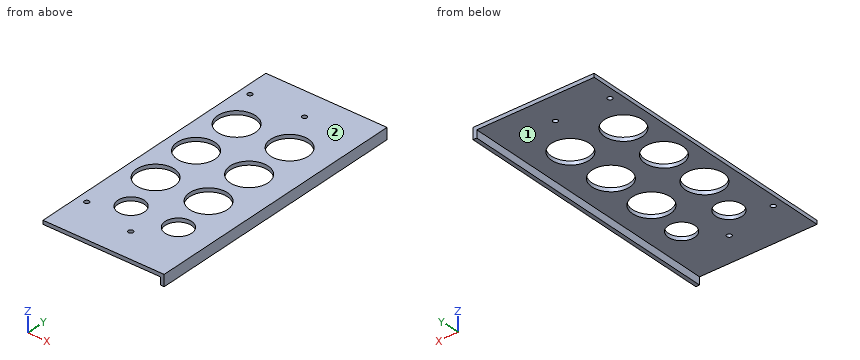
from build123d import *

# Parameters (mm, degrees)
SKETCH138_R           = 7
SKETCH138_R_2         = 10
EXTRUDE128_DEPTH      = 1
EXTRUDE128_DEPTH_BACK = 3
SKETCH117_R           = 1.28
EXTRUDE107_DEPTH      = 3
EXTRUDE104_DEPTH      = 143


with BuildPart() as extrude128:
    # Sketch138 → Extrude128 (new body, two sides)
    with BuildSketch(Plane(origin=(0, 0, -2), x_dir=(1, 0, 0), z_dir=(0, 0, -1))) as extrude128_sk:
        with Locations((28, -97)):
            Circle(SKETCH138_R)
        with Locations((53, -97)):
            Circle(SKETCH138_R)
        with Locations((22, -146)):
            Circle(SKETCH138_R_2)
        with Locations((50, -146)):
            Circle(SKETCH138_R_2)
        with Locations((22, -172)):
            Circle(SKETCH138_R_2)
        with Locations((50, -172)):
            Circle(SKETCH138_R_2)
        with Locations((22, -120)):
            Circle(SKETCH138_R_2)
        with Locations((50, -120)):
            Circle(SKETCH138_R_2)
    extrude(amount=EXTRUDE128_DEPTH)
    extrude(extrude128_sk.sketch, amount=-EXTRUDE128_DEPTH_BACK)


with BuildPart() as compound022:
    # Sketch117 → Extrude107 (new body)
    with BuildSketch(Plane(origin=(0, 0, 1), x_dir=(1, 0, 0), z_dir=(0, 0, -1))):
        with Locations((12, -88)):
            Circle(SKETCH117_R)
        with Locations((40, -82.25)):
            Circle(SKETCH117_R)
        with Locations((12, -192.75)):
            Circle(SKETCH117_R)
        with Locations((40, -193.75)):
            Circle(SKETCH117_R)
    extrude(amount=EXTRUDE107_DEPTH)

    # Compound022: union Extrude128
    add(extrude128.part)


with BuildPart() as hdmi002:
    # Sketch114 → Extrude104 (new body)
    with BuildSketch(Plane(origin=(0, 66, 0), x_dir=(-1, 0, 0), z_dir=(0, 1, 0))):
        Polygon((-7, -2), (-7, 0), (-71, 0), (-71, -6), (-69, -6), (-69, -2), align=None)
    extrude(amount=EXTRUDE104_DEPTH)

    # Cut013: cut Compound022
    add(compound022.part, mode=Mode.SUBTRACT)


solid = hdmi002.part
Can you work these out from the model? Positions are in its coordinate system, mm. Face numbers are marked on the shaded views. A direction names the side the tool comes from. Coordinates: 2 decimals unless noted, no trailing zeros. Loops run counter-clockwise (first coordinate to the right, second up) from the corner with the lowest first, then second, coordinate; pieces in that order, holes last. Notation, with made-up numbers: M -5,86 L 34,86 A11 ccw 34,94 Z; hole C 28.5,40.25 d11. An arc over 180 degrees is marked long. Return JSON: item names as keys, results as strings. Group by question number.
Item 1: Imagine slicing it at D-D (z = -0.9). Give the number of separate pieces and of enclosed holes in the cut face, and give its area (3 significant figures).
Item 2: On a 3-axis mill with a long thin cutter (end or side, diameter ignored), from which of +Z, -Z, +X, -X, +Y, -Y can I reach the whole of each face in a straight line? I mean the marked faces 1 and 2. Say none if no direction works.
Item 3: I'm going to push flat-ended pins straight in: pin 1 Ø1.2 at (y, z) = (121.5, -4.5) entering from -X; pin 2 Ø4 at (x, y) = (60.5, 98) entering from +Z; pin 3 Ø12 at (x, y) = (50, 120) entering from +Z; pin 4 Ø8 at (x, y) = (56, 140.5) entering from -Z. Where does each tip first touch, or does it pass through?
Item 4: If I drill on L1, parallel to X at y = 97, z = -1.5; L2, parallel to X at y = 172, z = -0.8; L3, parallel to Y at x = 53, z = -1.2, over which ranges is the centre line in solid material (lowest first)? Write a range as from..to.
Item 5: Imagine slicing it at B-B (y = 88). Please give me the cut outline in (x, z).
Item 6: Imagine slicing it at A-A (y = 120). Please give me the cut outline in (x, z).
Item 7: Imagine slicing it at C-C (x = 29.5). Please give me the cut outline in (y, z), and give its area (3 significant figures).
Verdict:
{
 "1": {"separate pieces": "1", "enclosed holes": "12", "area": "6,940 mm^2"},
 "2": {"face 1": "-Z, -X, +Y, -Y", "face 2": "+Z, +X, -X, +Y, -Y"},
 "3": {"pin 1": "stops at x = 69", "pin 2": "stops at z = 0", "pin 3": "passes through", "pin 4": "stops at z = -2"},
 "4": {"L1": "x = 7..21, 35..46, 60..71", "L2": "x = 7..12, 32..40, 60..71", "L3": "y = 66..90, 104..110.46, 129.54..136.46, 155.54..162.46, 181.54..209"},
 "5": {"outline": "M 7,-2 L 10.72,-2 L 10.72,0 L 7,0 Z; M 13.28,-2 L 69,-2 L 69,-6 L 71,-6 L 71,0 L 13.28,0 Z"},
 "6": {"outline": "M 7,-2 L 12,-2 L 12,0 L 7,0 Z; M 32,-2 L 40,-2 L 40,0 L 32,0 Z; M 60,-2 L 69,-2 L 69,-6 L 71,-6 L 71,0 L 60,0 Z"},
 "7": {"outline": "M 66,-2 L 90.16,-2 L 90.16,0 L 66,0 Z; M 103.84,-2 L 113.39,-2 L 113.39,0 L 103.84,0 Z; M 126.61,-2 L 139.39,-2 L 139.39,0 L 126.61,0 Z; M 152.61,-2 L 165.39,-2 L 165.39,0 L 152.61,0 Z; M 178.61,-2 L 209,-2 L 209,0 L 178.61,0 Z", "area": "179 mm^2"}
}
